Geometry: final body of the model. Coordinates: model frame, mm. Face numbers are marked on the shaded views. A direction names the side the tool comes from. Give positions to 0.01 mm unless a question says otherwise; leave off trailing zeros. Write each loop counter-clockwise with the first axis right and the second up, starting at its lowest first coordinate (ties: lowest second). Pieces come first, ordered by that corner, then holes. Notation, with made-up numbers: (-35.5, 38.25) -> (-4.5, 38.25) arc R24 ccw to (-4.5, 70.25) -> close; hole circle Ø10 at (22.25, 20). An arc over 180 degrees is marked (long way). Answer as a JSON object with one key per item and string values.
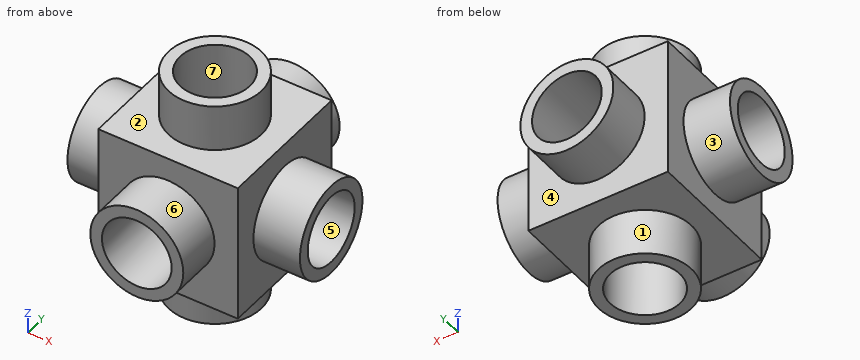
from build123d import *

# Parameters (mm, degrees)
F0_W      = 76.2
F0_H      = 76.2
F0_R      = 25.4
F1_DEPTH  = 38.1
F2_DEPTH  = 63.5
F3_R      = 25.4
F4_DEPTH  = 63.5
F5_R      = 25.4
F6_DEPTH  = 63.5
F7_R      = 19.05
F8_DEPTH  = 127.001
F9_R      = 19.05
F10_DEPTH = 127.001
F11_R     = 19.05
F12_DEPTH = 127.001
F13_W     = 50.8
F13_H     = 50.8
F14_DEPTH = 25.4


with BuildPart() as f1:
    # F0 (on Top) → F1 (new body, symmetric)
    with BuildSketch(Plane.XY):
        Rectangle(F0_W, F0_H)
        Circle(F0_R, mode=Mode.SUBTRACT)
    extrude(amount=F1_DEPTH, both=True)

    # F0 (on Top) → F2 (join, symmetric)
    with BuildSketch(Plane.XY):
        Circle(F0_R)
    extrude(amount=F2_DEPTH, both=True)

    # F3 (on Front) → F4 (join, symmetric)
    with BuildSketch(Plane.XZ):
        Circle(F3_R)
    extrude(amount=F4_DEPTH, both=True)

    # F5 (on Right) → F6 (join, symmetric)
    with BuildSketch(Plane.YZ):
        Circle(F5_R)
    extrude(amount=F6_DEPTH, both=True)

    # F7 (on face) → F8 (cut, through all)
    with BuildSketch(Plane.XY.offset(63.5)):
        Circle(F7_R)
    extrude(amount=-F8_DEPTH, mode=Mode.SUBTRACT)

    # F9 (on face) → F10 (cut, through all)
    with BuildSketch(Plane.XZ.offset(63.5)):
        Circle(F9_R)
    extrude(amount=-F10_DEPTH, mode=Mode.SUBTRACT)

    # F11 (on face) → F12 (cut, through all)
    with BuildSketch(Plane.YZ.offset(63.5)):
        Circle(F11_R)
    extrude(amount=-F12_DEPTH, mode=Mode.SUBTRACT)

    # F13 (on Front) → F14 (join, symmetric)
    with BuildSketch(Plane.XZ):
        Rectangle(F13_W, F13_H)
    extrude(amount=F14_DEPTH, both=True)


solid = f1.part
Q1. First-contact query: P1, Ø6, axis at x = -13.5, z = 31, coming from the -Y side; P2, Ø4, axis at y = -30.5, z = -41.5, coming from the +X side; P3, Ø23, axis at y = 0, z = 0, coming from the -X side; P4, Ø10, axis at x = 18, z = 34, coming from the +Y side. Flat tips, straight axial feed; report the tip coordinate or a pass-through.
Values:
{"P1": "y = -38.1", "P2": "through", "P3": "x = -25.4", "P4": "y = 38.1"}
Q2. Cut plane C-C (y = 21.5). Return the cut outline in (x, z).
Values:
{"outline": "(-63.5, -13.52) -> (-38.1, -13.52) -> (-38.1, -38.1) -> (-13.52, -38.1) -> (-13.52, -63.5) -> (13.52, -63.5) -> (13.52, -38.1) -> (38.1, -38.1) -> (38.1, -13.52) -> (63.5, -13.52) -> (63.5, 13.52) -> (38.1, 13.52) -> (38.1, 38.1) -> (13.52, 38.1) -> (13.52, 63.5) -> (-13.52, 63.5) -> (-13.52, 38.1) -> (-38.1, 38.1) -> (-38.1, 13.52) -> (-63.5, 13.52) -> close"}
Q3. Cut plane A-A (x = 32). Return the cut outline in (y, z).
Values:
{"outline": "(-38.1, -38.1) -> (38.1, -38.1) -> (38.1, 38.1) -> (-38.1, 38.1) -> close; hole circle Ø38.1 at (0, 0)"}
Q4. Material intervals for L1, parallel to Y at x = 0, z = 41; L2, parallel to Z at x = 0, y = 36, sorted ascending. Write a range as from..to.
Values:
{"L1": "-25.4..-19.05, 19.05..25.4", "L2": "-38.1..-19.05, 19.05..38.1"}
Q5. Set-up query: the marked faces 1, 2, 3 and 4. Return all of +Z, -Z, +X, -X, +Y, -Y with unobstructed straight access to the full face (end or side cutting, diameter ignored); none if empty.
Values:
{"face 1": "-Z", "face 2": "+Z", "face 3": "-X", "face 4": "+Y"}
Q6. Mould query, pull axis X, two halves, no side actions, for the marked faces 5, 6 and 7. Classes: pulls with the +X half, pulls with the -X half, needs draft (parallel to the pull), parting line crosses it, or undercut.
Values:
{"face 5": "needs draft", "face 6": "parting line crosses it", "face 7": "undercut"}
